Work out the finished part from the listing and answer in its coordinate system (mm). Face numbers are marked on the shaded views. A direction names the side the tool comes from. Coordinates: 2 decimals unless noted, no trailing zeros. Order: outer loops, then holes, each group sorted by start corner. A loop starts at its lowest first (then second) coordinate and runs counter-clockwise, first axis right, second up. Notation, with made-up numbers: (67.25, 28) - (126.25, 28) arc R31 cw to (126.25, 60) - close; hole circle Ø5 at (-27, 25). An arc over 180 degrees is marked (long way). Answer as a JSON object with one key per item and string values. Group by question number.
1) Find the intervals of material crossed by line 1 along Y through (x, z) = (0, 2.5); line 2 along Z through (x, y) = (1.5, -4); line 3 along Y through (x, z) = (2, 26.5), in increasing order.
2) A tool of negligible diameter and unlimited length cuts with its end or side. For the marked faces 4, 5, 6 and 7, from which of +Z, -Z, +X, -X, +Y, -Y can it reach the whole face along a straight path? Write none if from no direction.
3) The mould has two halves that part along Y. Classify the marked faces 1, 2 and 3: released by +Y, released by -Y, zero draft, split by the parting line, or undercut.
4) Section D-D (z = 23.25) is taken. Give the vertices of the cut face in (x, y).
5) Each of these flat-tipped pins is pushed along its axis until it touches: P1, Ø4, axis at x = 4.5, z = 9.5, coming from the -Y side; P2, Ø1, axis at x = 2.5, y = 3, coming from the -Z side; P3, Ø2, axis at x = 1.5, z = 22, coming from the +Y side. Where does it stop, or does it pass through?
6) Section B-B (y = -4.5) is taken. Give the vertices of the cut face in (x, z).
7) Section A-A (z = 10.25) is taken. Give the vertices of the cut face in (x, y), plus the area to 3 significant figures.
8) Section C-C (x = 1.25) is taken. Give the vertices of the cut face in (y, z).
from build123d import *

# Parameters (mm, degrees)
F0_R     = 6.5
F0_R_2   = 5
F1_DEPTH = 8
F2_R     = 6.5
F3_DEPTH = 11
F4_R     = 6.5
F5_DEPTH = 0.5
F6_W     = 6.929646
F6_H     = 6.929646
F7_DEPTH = 10


with BuildPart() as f1:
    # F0 (on Top) → F1 (new body)
    with BuildSketch(Plane.XY):
        Circle(F0_R)
        Circle(F0_R_2, mode=Mode.SUBTRACT)
    extrude(amount=F1_DEPTH)

    # F2 (on face) → F3 (join)
    with BuildSketch(Plane.XY.offset(8)):
        Circle(F2_R)
        Polygon((4.755283, 1.545085), (2.938926, -4.045085), (-2.938926, -4.045085), (-4.755283, 1.545085), (0, 5), align=None, mode=Mode.SUBTRACT)
    extrude(amount=F3_DEPTH)

    # F4 (on face) → F5 (join)
    with BuildSketch(Plane.XY.offset(19)):
        Circle(F4_R)
    extrude(amount=F5_DEPTH)

    # F6 (on face) → F7 (join)
    with BuildSketch(Plane.XY.offset(19.5)):
        Rectangle(F6_W, F6_H)
    extrude(amount=F7_DEPTH)


solid = f1.part
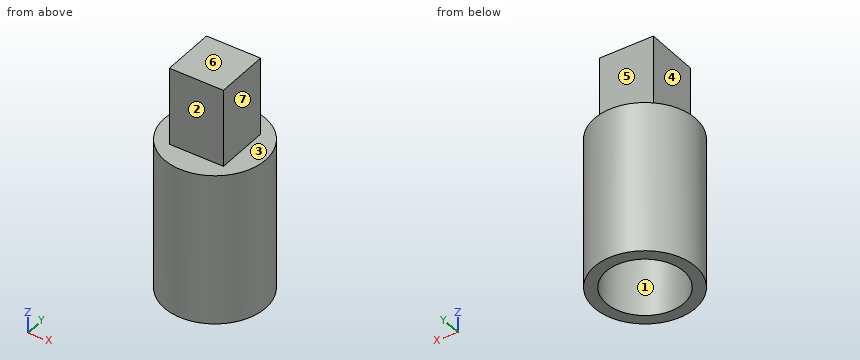
Report:
{
 "1": {"line 1": "y = -6.5 to -5, 5 to 6.5", "line 2": "z = 19 to 19.5", "line 3": "y = -3.46 to 3.46"},
 "2": {"face 4": "+Z, -X, +Y, -Y", "face 5": "+Z, +X, -X, +Y", "face 6": "+Z, +X, -X, +Y, -Y", "face 7": "+Z, +X, +Y, -Y"},
 "3": {"face 1": "undercut", "face 2": "released by -Y", "face 3": "zero draft"},
 "4": {"outline": "(-3.46, -3.46) - (3.46, -3.46) - (3.46, 3.46) - (-3.46, 3.46) - close"},
 "5": {"P1": "stops at y = -6", "P2": "stops at z = 8", "P3": "stops at y = 3.46"},
 "6": {"outline": "(-4.69, 0) - (-2.18, 0) - (-2.18, 8) - (2.18, 8) - (2.18, 0) - (4.69, 0) - (4.69, 19.5) - (-4.69, 19.5) - close"},
 "7": {"outline": "circle Ø13 at (0, 0); hole (-4.76, 1.55) - (-2.94, -4.05) - (2.94, -4.05) - (4.76, 1.55) - (0, 5) - close", "area": "73.3 mm²"},
 "8": {"outline": "(-6.38, 0) - (-4.84, 0) - (-4.84, 8) - (-4.05, 8) - (-4.05, 19) - (4.09, 19) - (4.09, 8) - (4.84, 8) - (4.84, 0) - (6.38, 0) - (6.38, 19.5) - (3.46, 19.5) - (3.46, 29.5) - (-3.46, 29.5) - (-3.46, 19.5) - (-6.38, 19.5) - close"}
}
